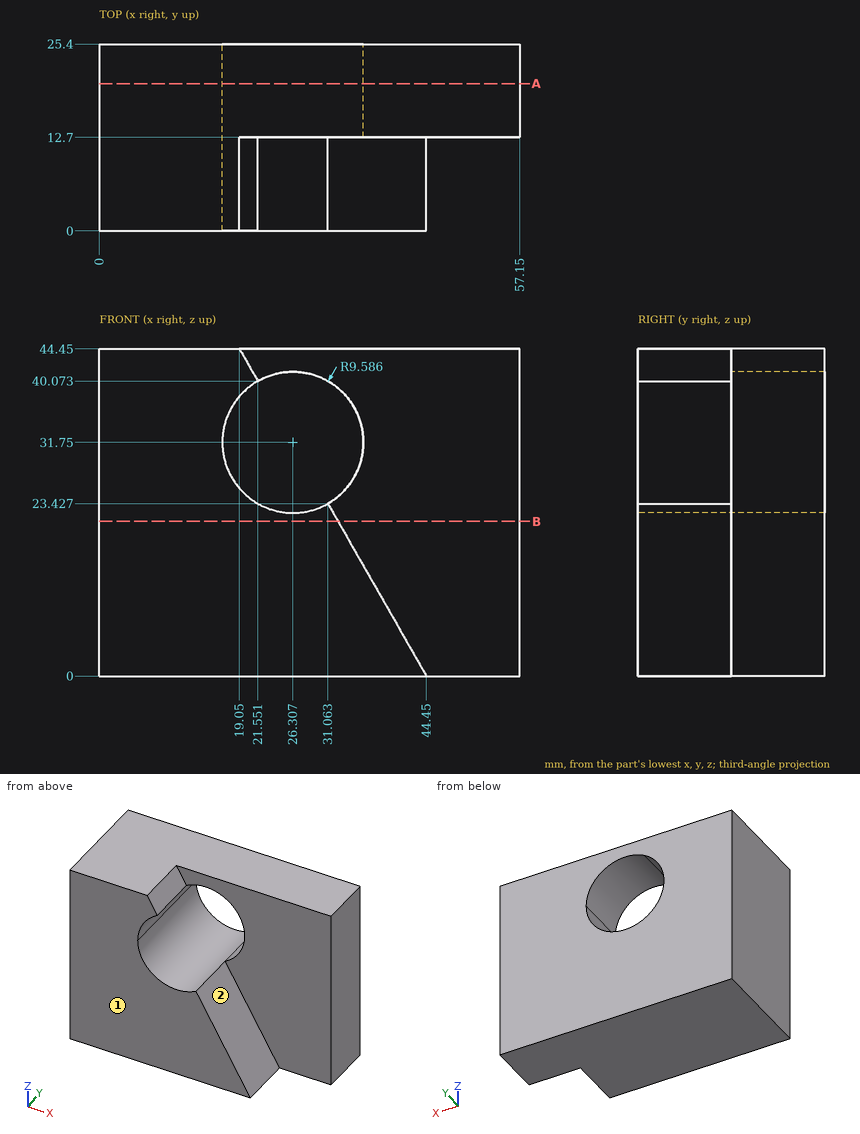
For this review, use the dimensioned drawing (mm, ordinates from the lowest corner) and the shaded views. A direction names the side the tool comes from. Give positions to 0.01 mm unless a question says otherwise; leave off trailing zeros. Order: outer loops, then holes, each group sorted by start corner. A loop starts at its lowest first (then second) coordinate and runs counter-clockwise, first axis right, second up. Notation, with made-up numbers: (-38.5, 56) - (-33.5, 56) arc R24 cw to (-33.5, 82) - close; hole circle Ø3 at (76.25, 1). An arc over 180 degrees is marked (long way). Use a Markdown table: item, result. Add a question column.
(1) Wall thickness on probe 1 along Y at (x, z) = (49, 36.5); probe 2 along Z at (x, y) = (25.5, 22.75); probe 3 along X at (y, z) = (23.25, 37.5): over which ranges is each line inside the solid? List them lowest first. Write a range as [from, to].
(2) Add section B-B on z = 21. Give the boundary of the cut face in (x, y), then the cut area to 3 significant figures.
(3) Machinability: for the marked faces 1 and 2, which of the approach directions +Z, -Z, +X, -X, +Y, -Y give a long, thin tool a straight path to every point of the face, cutting with its end or side? Answer none if there is none.
(4) Add section A-A on y = 20. Give the boundary of the cut face in (x, z).
Report:
| question | item | result |
|---|---|---|
| 1 | probe 1 | y = [12.7, 25.4] |
| 1 | probe 2 | z = [0, 22.2], [41.3, 44.45] |
| 1 | probe 3 | x = [0, 18.64], [33.98, 57.15] |
| 2 | outline | (0, 0) - (32.45, 0) - (32.45, 12.7) - (57.15, 12.7) - (57.15, 25.4) - (0, 25.4) - close |
| 2 | area | 1,140 mm² |
| 3 | face 1 | +Z, -Z, +X, -X, -Y |
| 3 | face 2 | +Z, +X, -Y |
| 4 | outline | (0, 0) - (57.15, 0) - (57.15, 44.45) - (0, 44.45) - close; hole circle Ø19.17 at (26.31, 31.75) |
